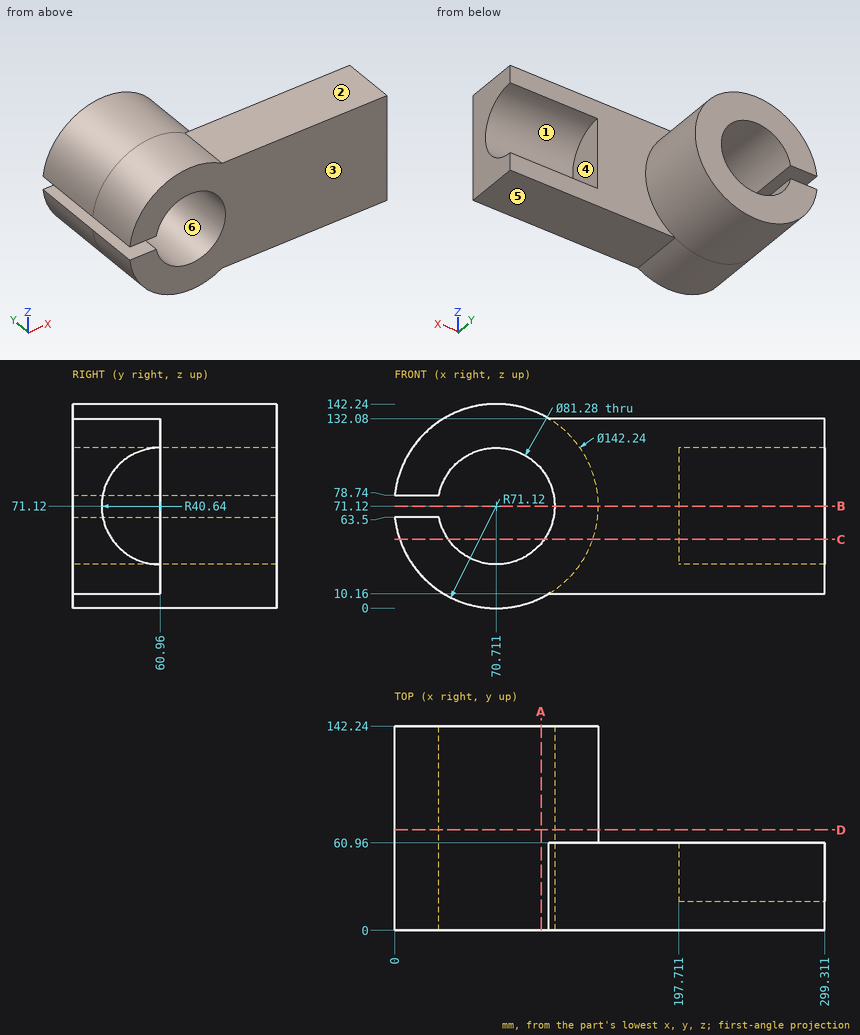
Job drawing, mm, ordinate dimensions from the low corner. One solid piece. A direction names the side the tool comes from. Round coordinates to 2 decimals unless told otherwise and drop trailing zeros. Loops run counter-clockwise (first coordinate to the right, second up) from the corner with the lowest first, then second, coordinate; pieces in that order, holes last.
Item 1: Cut at A-A, the plane x = 102. Give the cut face in (y, z) (1 decimal), then the cut area to 3 significant figures.
Item 2: Mould opens along X. For the marked faces 4, 5 and 6 say: +X half, -X half, draft (parallel to the pull), parting line (faces both ways), or undercut.
Item 3: Cut at B-B, the plane z = 71.12. Give the cut face in (x, y).
Item 4: Cut at C-C, the plane z = 48. Give the cut face in (x, y), then the cut area to 3 significant figures.
Item 5: 3-axis set-ups, long thin cutter, end or side, ignore diameter. For the marked faces 1, 2 and 3: which of +Z, -Z, +X, -X, +Y, -Y reach the whole face in a straight line?
Item 6: Drop flat-ended pins along their axis: P1, Ø12, axis at y = 88, z = 41.5, coming from the +X side; P2, Ø1, axis at x = 82, y = 127.5, coming from the -Z side; P3, Ø8, axis at x = 224.5, z = 78.5, coming from the +Y side; P4, Ø12, axis at x = 220.5, y = 68, coming from the -Z side. Give the stop position or say it passes through.
Item 7: Drill centre lines: line 1 (Y direction, x = 145, z = 13); line 2 (X direction, y = 98, z = 71.12); line 3 (Z direction, x = 37, y = 108.5) (1 decimal). Where is each one in solid material? Low to high.
Item 8: Cut at D-D, the plane y = 70. Give the cut face in (x, z), then the cut area to 3 significant figures.
A:
1. outline: (0, 7.3) - (142.2, 7.3) - (142.2, 45.2) - (0, 45.2) - close; (0, 97.1) - (142.2, 97.1) - (142.2, 135) - (0, 135) - close
1. area: 10,800 mm2
2. face 4: +X half
2. face 5: draft
2. face 6: undercut
3. outline: (111.35, 0) - (299.31, 0) - (299.31, 20.32) - (197.71, 20.32) - (197.71, 60.96) - (141.83, 60.96) - (141.83, 142.24) - (111.35, 142.24) - close
4. outline: (3.45, 0) - (37.29, 0) - (37.29, 142.24) - (3.45, 142.24) - close; (104.13, 0) - (299.31, 0) - (299.31, 27.54) - (197.71, 27.54) - (197.71, 60.96) - (137.97, 60.96) - (137.97, 142.24) - (104.13, 142.24) - close
4. area: 16,100 mm2
5. face 1: +X, +Y
5. face 2: +Z, +X, +Y, -Y
5. face 3: +Z, -Z, +X, -X, -Y
6. P1: stops at x = 137.79
6. P2: stops at z = 0.82
6. P3: stops at y = 21.95
6. P4: passes through
7. line 1: y = 0 to 60.96
7. line 2: x = 111.35 to 141.83
7. line 3: z = 8.5 to 48.4, 93.8 to 133.7
8. outline: (0, 63.5) arc R71.12 ccw (long way) to (0, 78.74) - (30.79, 78.74) arc R40.64 cw (long way) to (30.79, 63.5) - close
8. area: 10,200 mm2
